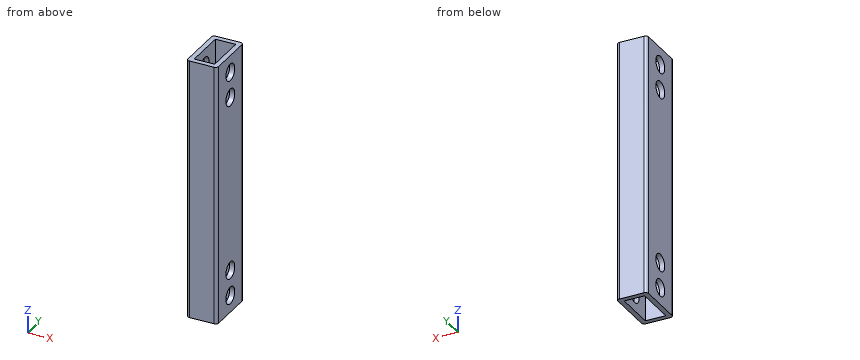
```python
from build123d import *

# Parameters (mm, degrees)
SKETCH1_W         = 18
SKETCH1_H         = 30
SKETCH1_W_2       = 12
SKETCH1_H_2       = 24
BODY_DEPTH        = 153.15701543
SKETCH2_R         = 5
MOUNT_HOLES_DEPTH = 155.938927889
CORNER_FILLETS_R  = 1.8


with BuildPart() as part:
    # Sketch1 → Body (new body)
    with BuildSketch(Plane.XY):
        Rectangle(SKETCH1_W, SKETCH1_H)
        Rectangle(SKETCH1_W_2, SKETCH1_H_2, mode=Mode.SUBTRACT)
    extrude(amount=BODY_DEPTH)

    # Sketch2 → Mount Holes (cut, through all)
    with BuildSketch(Plane(origin=(9, 0, 0), x_dir=(0, 0, -1), z_dir=(1, 0, 0))):
        with Locations((-143.15701543, 0)):
            Circle(SKETCH2_R)
        with Locations((-128.15701543, 0)):
            Circle(SKETCH2_R)
        with Locations(Location((-25, 0, 0), (0, 0, 180))):
            Circle(SKETCH2_R)
        with Locations(Location((-10, 0, 0), (0, 0, 180))):
            Circle(SKETCH2_R)
    extrude(amount=-MOUNT_HOLES_DEPTH, mode=Mode.SUBTRACT)

    # Corner Fillets
    corner_fillets_edges = [part.edges().sort_by_distance(p)[0] for p in [
        (-9, 15, 76.578507715),
        (9, 15, 76.578507715),
        (9, -15, 76.578507715),
        (-9, -15, 76.578507715),
    ]]
    fillet(corner_fillets_edges, radius=CORNER_FILLETS_R)


solid = part.part
```
Input: part model. Units: mm. Frame: model coordinates. Round coordinates to 2 decimals unless told otherwise and drop trailing zeros. Loops run counter-clockwise (first coordinate to the right, second up) from the corner with the lowest first, then second, coordinate; pieces in that order, holes last. Notation, with made-up numbers: (80.25, 43) -> (90.25, 43) arc R23 cw to (90.25, 62) -> close; hole circle Ø2 at (23.5, 38). An arc over 180 degrees is marked (long way). One line per item, written item: value.
(1) Section B-B (z = 85). Return the cut outline in (x, y).
Geometry check:
outline: (-9, -13.2) arc R1.8 ccw to (-7.2, -15) -> (7.2, -15) arc R1.8 ccw to (9, -13.2) -> (9, 13.2) arc R1.8 ccw to (7.2, 15) -> (-7.2, 15) arc R1.8 ccw to (-9, 13.2) -> close; hole (-6, -12) -> (6, -12) -> (6, 12) -> (-6, 12) -> close
(2) Material intervals for line 1 (X direction, y = 6.25, z = 30); line 2 (Y direction, x = 3.5, z = 89); line 3 (Y direction, x = -7.75, z = 25), sorted ascending. Write a range as [from, to].
Geometry check:
line 1: [-9, -6], [6, 9]
line 2: [-15, -12], [12, 15]
line 3: [-14.91, -5], [5, 14.91]
(3) Section A-A (y = 6.5). Return the cut outline in (x, z), plus the area to 3 significant figures.
Geometry check:
outline: (-9, 0) -> (-6, 0) -> (-6, 153.16) -> (-9, 153.16) -> close; (6, 0) -> (9, 0) -> (9, 153.16) -> (6, 153.16) -> close
area: 919 mm2
(4) Section D-D (z = 13.5). Return the cut outline in (x, y), plus the area to 3 significant figures.
Geometry check:
outline: (-9, -13.2) arc R1.8 ccw to (-7.2, -15) -> (7.2, -15) arc R1.8 ccw to (9, -13.2) -> (9, -3.57) -> (6, -3.57) -> (6, -12) -> (-6, -12) -> (-6, -3.57) -> (-9, -3.57) -> close; (-9, 3.57) -> (-6, 3.57) -> (-6, 12) -> (6, 12) -> (6, 3.57) -> (9, 3.57) -> (9, 13.2) arc R1.8 ccw to (7.2, 15) -> (-7.2, 15) arc R1.8 ccw to (-9, 13.2) -> close
area: 206 mm2
(5) Section C-C (x = 1.5). Return the cut outline in (y, z).
Geometry check:
outline: (-15, 0) -> (-12, 0) -> (-12, 153.16) -> (-15, 153.16) -> close; (12, 0) -> (15, 0) -> (15, 153.16) -> (12, 153.16) -> close
